Could you check a few things on this model? Use its own coordinates, in mm. Face numbers are marked on the shaded views. A direction names the side the tool comes from. Round coordinates to 2 decimals unless told otherwise and drop trailing zeros. Loops run counter-clockwise (first coordinate to the right, second up) from the corner with the lowest first, then second, coordinate; pieces in that order, holes last. Notation, with made-up numbers: (-28, -23.5) -> (-15, -23.5) arc R13 ccw to (-15, -14.5) -> close; hole circle Ø5 at (47.25, 15). An arc over 180 degrees is marked (long way). One line per item, written item: value.
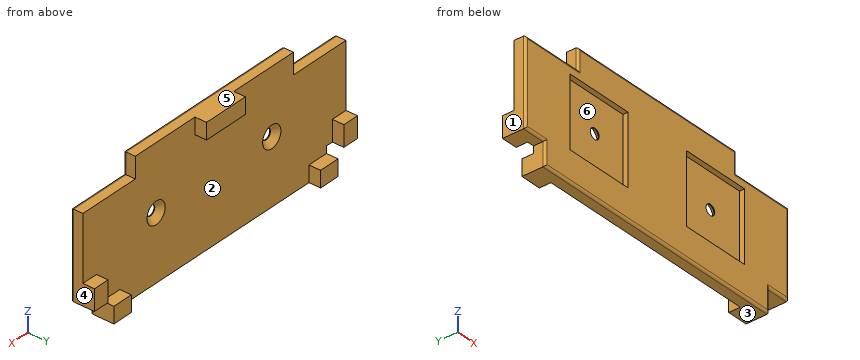
from build123d import *

# Parameters (mm, degrees)
SKETCH1_W                                     = 135.4
SKETCH1_H                                     = 55.7
BOSS_EXTRUDE1_DEPTH                           = 5
SKETCH2_W                                     = 20
SKETCH2_H                                     = 7
BOSS_EXTRUDE2_DEPTH                           = 5
SKETCH3_W                                     = 27
SKETCH3_H                                     = 9
CUT_EXTRUDE1_DEPTH                            = 74.375149063
CSK_FOR_M4_COUNTERSUNK_FLAT_HEAD1_D           = 4.5
CSK_FOR_M4_COUNTERSUNK_FLAT_HEAD1_CSINK_D     = 9.4
CSK_FOR_M4_COUNTERSUNK_FLAT_HEAD1_CSINK_ANGLE = 90
SKETCH7_W                                     = 30
SKETCH7_H                                     = 30
CUT_EXTRUDE2_DEPTH                            = 2.2
SKETCH9_W                                     = 10
SKETCH9_H                                     = 10
CUT_EXTRUDE5_DEPTH                            = 74.88445371
FILLET1_R                                     = 1


with BuildPart() as part:
    # Sketch1 → Boss-Extrude1 (new body)
    with BuildSketch(Plane(origin=(0, 0, 0), x_dir=(1, 0, 0), z_dir=(0, 1, 0))):
        Rectangle(SKETCH1_W, SKETCH1_H)
    extrude(amount=BOSS_EXTRUDE1_DEPTH)

    # Sketch2 → Boss-Extrude2 (add)
    with BuildSketch(Plane(origin=(0, 5, 0), x_dir=(1, 0, 0), z_dir=(0, 1, 0))):
        Polygon((-60.7, 20.85), (-48.7, 20.85), (-48.7, 27.85), (-67.7, 27.85), (-67.7, 8.85), (-60.7, 8.85), align=None)
        with Locations((0, -24.35)):
            Rectangle(SKETCH2_W, SKETCH2_H)
        Polygon((67.7, 27.85), (48.7, 27.85), (48.7, 20.85), (60.7, 20.85), (60.7, 8.85), (67.7, 8.85), align=None)
    extrude(amount=BOSS_EXTRUDE2_DEPTH)

    # Sketch3 → Cut-Extrude1 (cut, through all)
    with BuildSketch(Plane(origin=(0, 5, 0), x_dir=(1, 0, 0), z_dir=(0, 1, 0))):
        with Locations((-54.2, -23.35)):
            Rectangle(SKETCH3_W, SKETCH3_H)
    cut_extrude1 = extrude(amount=-CUT_EXTRUDE1_DEPTH, mode=Mode.SUBTRACT)

    # Mirror1: Cut-Extrude1 across plane
    add(cut_extrude1.mirror(Plane(origin=(0, 0, 0), x_dir=(0, 0, 1), z_dir=(1, 0, 0))), mode=Mode.SUBTRACT)

    # CSK for M4 Countersunk Flat Head1 (through all)
    with Locations(Plane(origin=(-29.527844293, 5, 0), x_dir=(0, 0, 1), z_dir=(0, 1, 0))):
        with Locations((0, 0), (0, 59.527844293)):
            CounterSinkHole(CSK_FOR_M4_COUNTERSUNK_FLAT_HEAD1_D / 2, CSK_FOR_M4_COUNTERSUNK_FLAT_HEAD1_CSINK_D / 2, counter_sink_angle=CSK_FOR_M4_COUNTERSUNK_FLAT_HEAD1_CSINK_ANGLE)

    # Sketch7 → Cut-Extrude2 (cut)
    with BuildSketch(Plane.XZ):
        with Locations((-30, 0)):
            Rectangle(SKETCH7_W, SKETCH7_H)
        with Locations((30, 0)):
            Rectangle(SKETCH7_W, SKETCH7_H)
    extrude(amount=-CUT_EXTRUDE2_DEPTH, mode=Mode.SUBTRACT)

    # Sketch9 → Cut-Extrude5 (cut, through all)
    with BuildSketch(Plane(origin=(0, 10, 0), x_dir=(1, 0, 0), z_dir=(0, 1, 0))):
        with Locations((62.7, 22.85)):
            Rectangle(SKETCH9_W, SKETCH9_H)
    cut_extrude5 = extrude(amount=-CUT_EXTRUDE5_DEPTH, mode=Mode.SUBTRACT)

    # Mirror2: Cut-Extrude5 across plane
    add(cut_extrude5.mirror(Plane(origin=(0, 0, 0), x_dir=(0, 0, 1), z_dir=(1, 0, 0))), mode=Mode.SUBTRACT)

    # Fillet1
    fillet1_edges = [part.edges().sort_by_distance(p)[0] for p in [
        (0, 0, -27.85),
        (62.7, 0, -17.85),
        (57.7, 0, -22.85),
        (-67.7, 0, 0.5),
        (-57.7, 0, -22.85),
        (-62.7, 0, -17.85),
        (0, 0, 27.85),
        (-54.2, 0, 18.85),
        (-40.7, 0, 23.35),
        (67.7, 0, 0.5),
        (40.7, 0, 23.35),
        (54.2, 0, 18.85),
    ]]
    fillet(fillet1_edges, radius=FILLET1_R)


solid = part.part
(1) If we section it at C-C, the plane x = 30: Please give me the cut outline in (y, z), then the cut area to 3 significant figures.
Recorded:
outline: (0, -26.85) arc R1 ccw to (1, -27.85) -> (5, -27.85) -> (5, -4.7) -> (2.55, -2.25) -> (2.2, -2.25) -> (2.2, -15) -> (0, -15) -> close; (0, 15) -> (2.2, 15) -> (2.2, 2.25) -> (2.55, 2.25) -> (5, 4.7) -> (5, 27.85) -> (1, 27.85) arc R1 ccw to (0, 26.85) -> close
area: 193 mm²
(2) Thinking about a two-plate mould opening in X: for the marked faces 1, 2, 3 and 4, which applies, released by +X, released by -X, zero draft, split by the parting line, or undercut?
Recorded:
face 1: released by -X
face 2: undercut
face 3: zero draft
face 4: released by +X
(3) If I drill on L1, parallel to X at y = 2.4, z = 0; L2, parallel to X at y = 6, z = -24.5; L3, parallel to Y at x = -51, z = -3.5, over which ranges is the centre line in solid material (lowest first)?
Recorded:
L1: -67.7 to -31.78, -27.28 to 27.75, 32.25 to 67.7
L2: -57.7 to -48.7, 48.7 to 57.7
L3: 0 to 5
(4) If we section it at B-B, the plane y = 8: Please give me the cut outline in (x, z), then the cut area to 3 significant figures.
Recorded:
outline: (-67.7, -17.85) -> (-60.7, -17.85) -> (-60.7, -8.85) -> (-67.7, -8.85) -> close; (-57.7, -27.85) -> (-48.7, -27.85) -> (-48.7, -20.85) -> (-57.7, -20.85) -> close; (-10, 20.85) -> (10, 20.85) -> (10, 27.85) -> (-10, 27.85) -> close; (48.7, -27.85) -> (57.7, -27.85) -> (57.7, -20.85) -> (48.7, -20.85) -> close; (60.7, -17.85) -> (67.7, -17.85) -> (67.7, -8.85) -> (60.7, -8.85) -> close
area: 392 mm²
(5) For the marked faces 5 and 6, which set-ups out of +Z, -Z, +X, -X, +Y, -Y let a thin tool reach every point of the face, with its end or its side?
Recorded:
face 5: +Z, +X, -X, +Y, -Y
face 6: -Y
(6) I'm going to push flat-ended pins straight in: pin 1 Ø5.5 at (x, y) = (3.5, 8.5) entering from -Z; pin 2 Ø5.5 at (y, z) = (7.5, 23) entering from +X; pin 3 Ø4 at (x, y) = (-63.5, 8) entering from +Z. Where does each tip first touch, or does it pass through?
Recorded:
pin 1: z = 20.85
pin 2: x = 40.7
pin 3: z = -8.85
(7) If we section it at A-A, the plane z = 0: Please give me the cut outline in (x, y), then the cut area to 3 significant figures.
Recorded:
outline: (-67.7, 1) arc R1 ccw to (-66.7, 0) -> (-45, 0) -> (-45, 2.2) -> (-31.78, 2.2) -> (-31.78, 2.55) -> (-34.23, 5) -> (-67.7, 5) -> close; (-27.28, 2.2) -> (-15, 2.2) -> (-15, 0) -> (15, 0) -> (15, 2.2) -> (27.75, 2.2) -> (27.75, 2.55) -> (25.3, 5) -> (-24.83, 5) -> (-27.28, 2.55) -> close; (32.25, 2.2) -> (45, 2.2) -> (45, 0) -> (66.7, 0) arc R1 ccw to (67.7, 1) -> (67.7, 5) -> (34.7, 5) -> (32.25, 2.55) -> close
area: 507 mm²
(8) If we section it at D-D, the plane z = 24: Please give me the cut outline in (x, y), then the cut area to 3 significant figures.
Recorded:
outline: (-40.7, 1) arc R1 ccw to (-39.7, 0) -> (39.7, 0) arc R1 ccw to (40.7, 1) -> (40.7, 5) -> (10, 5) -> (10, 10) -> (-10, 10) -> (-10, 5) -> (-40.7, 5) -> close
area: 507 mm²
